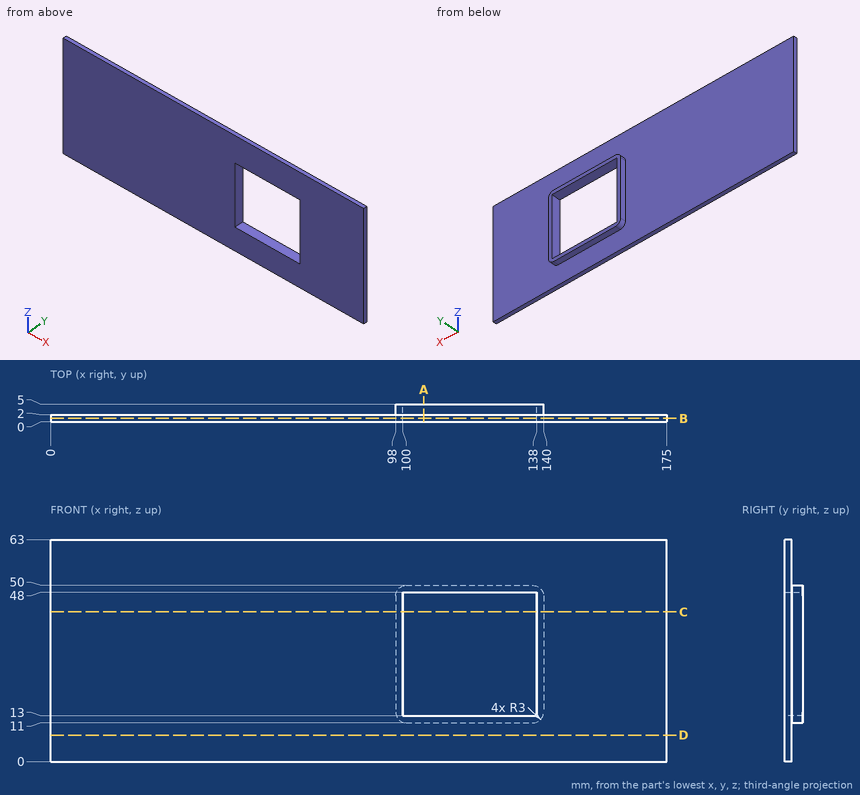
The figure shows three views and two pictorial views of one solid part (mm, origin at its lowest corner). Answer the questions. Give positions to 0.01 mm unless a question says otherwise; leave off trailing zeros. Write each loop counter-clockwise with the first axis right and the second up, starting at its lowest first coordinate (ties: lowest second). Pieces come first, ordered by that corner, then holes. Notation, with made-up numbers: (25.5, 76) - (81.5, 76) arc R35 cw to (81.5, 113) - close; hole circle Ø5 at (11, 79.25). An arc over 180 degrees is marked (long way). Use one line per item in the form item = value. Start each with the question number.
1) Find section C-C on z = 42.5. Determine the outline of the cut face in (x, y).
2) Find section D-D on z = 7.5. Determine the outline of the cut face in (x, y).
3) Find section A-A on x = 106. Determine the outline of the cut face in (y, z).
4) Consider line 1 along Z through (x, y) = (128.5, 3.35); line 2 along X through (y, z) = (2.8, 29); line 3 along Z through (x, y) = (114.5, 0.3). Determine where each line is inside the solid, lowest interval first. Write a range as from..to.
5) Flat-ended cylindrical pins translate along their axes: pin 1 Ø8 at (x, z) = (155.5, 33.5) entering from +Y; pin 2 Ø2 at (y, z) = (4, 38) entering from -X; pin 3 Ø1 at (x, y) = (64.5, 3.5) entering from -Z; pin 4 Ø0.9 at (x, y) = (127.5, 3) entering from +Z. Find the tip coordinate at first contact, or state that the pin passes through.
6) Find section B-B on y = 0.9. Determine the outline of the cut face in (x, z).
Geometry results:
q1.outline = (0, 0) - (100, 0) - (100, 5) - (98, 5) - (98, 2) - (0, 2) - close; (138, 0) - (175, 0) - (175, 2) - (140, 2) - (140, 5) - (138, 5) - close
q2.outline = (0, 0) - (175, 0) - (175, 2) - (0, 2) - close
q3.outline = (0, 0) - (2, 0) - (2, 11) - (5, 11) - (5, 13) - (0, 13) - close; (0, 48) - (5, 48) - (5, 50) - (2, 50) - (2, 63) - (0, 63) - close
q4.line_1 = 11..13, 48..50
q4.line_2 = 98..100, 138..140
q4.line_3 = 0..13, 48..63
q5.pin_1 = 2
q5.pin_2 = 98
q5.pin_3 = through
q5.pin_4 = 50
q6.outline = (0, 0) - (175, 0) - (175, 63) - (0, 63) - close; hole (100, 13) - (138, 13) - (138, 48) - (100, 48) - close
